from build123d import *

# Parameters (mm, degrees)
SKETCH_R     = 11.25
SKETCH_R_2   = 8.25
PAD_DEPTH    = 50
SKETCH001_R  = 11.25
PAD001_DEPTH = 100
POCKET_DEPTH = 25


with BuildPart() as part:
    # Sketch → Pad (new body)
    with BuildSketch(Plane.XY):
        Circle(SKETCH_R)
        Circle(SKETCH_R_2, mode=Mode.SUBTRACT)
    extrude(amount=PAD_DEPTH)

    # Sketch001 (on Face3 of Pad) → Pad001 (join)
    with BuildSketch(Plane(origin=(0, 0, 0), x_dir=(1, 0, 0), z_dir=(0, 0, -1))):
        Circle(SKETCH001_R)
    extrude(amount=PAD001_DEPTH)

    # Sketch002 (on Face3 of Pad001) → Pocket (cut)
    with BuildSketch(Plane.XY.offset(50)):
        with BuildLine():
            ThreePointArc((8.124664, 1.432597), (0, 8.25), (-8.124664, 1.432597))
            Line((-11.079087, 1.953542), (-8.124664, 1.432597))
            ThreePointArc((11.079087, 1.953542), (0, 11.25), (-11.079087, 1.953542))
            Line((11.079087, 1.953542), (8.124664, 1.432597))
        make_face()
    extrude(amount=-POCKET_DEPTH, mode=Mode.SUBTRACT)


solid = part.part
Work out the finished part from the listing and answer in its coordinate system (mm). A direction names the side the tool comes from. Give positions to 0.01 mm unless a question says otherwise; leave off trailing zeros. Order: outer loops, then holes, each group sorted by start corner. A loop starts at its lowest first (then second) coordinate and runs counter-clockwise, first axis right, second up. Notation, with made-up numbers: M -16,57.5 L 33,57.5 A27 cw 33,80.5 Z; hole C 15,35.5 d1. An arc over 180 degrees is marked long. Return JSON: item names as keys, results as strings.
Q1. Find section C-C, the plane z = -26. Write down the section's boundary in (x, y).
Answer below:
{"outline": "C 0,0 d22.5"}
Q2. Each of these flat-tipped pins is pushed along its axis until it touches: pin 1 (3 mm diameter, centred on x = -3, z = -42, fed in from -Y); pin 2 (8 mm diameter, centred on y = -7, z = -4, fed in from -X); pin 3 (3 mm diameter, centred on x = 2, z = 27, fed in from -Y). Where does it stop, or does it pass through?
Answer below:
{"pin 1": "stops at y = -11.15", "pin 2": "stops at x = -10.84", "pin 3": "stops at y = -11.24"}
Q3. The mould has two halves that part along Y. Classify faces 1 (the face through (0, 0, 0)), 2 (the face through (-1.465, -11.154, -23.95)), 3 (the face through (0, -9, 50)), 4 (the face through (-1.788, -8.054, 19.094)): pulls with the +Y half, pulls with the -Y half, needs draft (parallel to the pull), parting line crosses it, or undercut.
Answer below:
{"face 1": "undercut", "face 2": "parting line crosses it", "face 3": "needs draft", "face 4": "undercut"}
Q4. Find the intervals of material crossed by line 1 along Y through (x, z) = (0, 16.5); line 2 along Z through (x, y) = (5, 6.25), in increasing order. Write a range as [from, to].
Answer below:
{"line 1": "y = [-11.25, -8.25], [8.25, 11.25]", "line 2": "z = [-100, 0]"}
Q5. Find section A-A, the plane y = 0. Write down the section's boundary in (x, z).
Answer below:
{"outline": "M -11.25,-100 L 11.25,-100 L 11.25,50 L 8.25,50 L 8.25,0 L -8.25,0 L -8.25,50 L -11.25,50 Z"}
Q6. Find section D-D, the plane z = 28.5. Write down the section's boundary in (x, y), and give its area (3 significant figures).
Answer below:
{"outline": "M -11.08,1.95 A11.25 ccw long 11.08,1.95 L 8.12,1.43 A8.25 cw long -8.12,1.43 Z", "area": "102 mm^2"}
Q7. Which of the six approach directions +Z, -Z, +X, -X, +Y, -Y give full straight-line access (tool end or side, diameter ignored) to faces 5 (the face through (-9.623, 1.697, 37.675)), 6 (the face through (0, 0, -100))?
Answer below:
{"face 5": "+Z, +Y", "face 6": "-Z, +X, -X, +Y, -Y"}
Q8. Find section B-B, the plane x = 0. Write down the section's boundary in (y, z), and give its area (4 significant figures).
Answer below:
{"outline": "M -11.25,-100 L 11.25,-100 L 11.25,25 L 8.25,25 L 8.25,0 L -8.25,0 L -8.25,50 L -11.25,50 Z", "area": "2,475 mm^2"}
